```python
from build123d import *

# Parameters (mm, degrees)
SKETCH_1_R      = 2
SKETCH_1_R_2    = 1.65
EXTRUDE_1_DEPTH = 300
FILLET_1_R      = 0.2


with BuildPart() as part:
    # 草图1 → 凸台-拉伸1 (new body)
    with BuildSketch(Plane(origin=(0, 0, 0), x_dir=(1, 0, 0), z_dir=(0, 1, 0))):
        with BuildLine():
            Line((-9.5, 10), (-2.15, 10))
            Line((-2.15, 10), (-2.15, 8.7))
            Line((-2.15, 8.7), (-4, 8.7))
            Line((-4, 8.7), (-4, 4.7))
            Line((-4, 4.7), (-2.15, 4.7))
            Line((-2.15, 4.7), (-2.15, 2.9))
            Line((-2.15, 2.9), (0, 2.9))
            Line((0, 2.9), (2.15, 2.9))
            Line((2.15, 2.9), (2.15, 4.7))
            Line((2.15, 4.7), (4, 4.7))
            Line((4, 4.7), (4, 8.7))
            Line((4, 8.7), (2.15, 8.7))
            Line((2.15, 8.7), (2.15, 10))
            Line((2.15, 10), (9.5, 10))
            ThreePointArc((9.5, 10), (9.853553391, 9.853553391), (10, 9.5))
            Line((10, 9.5), (10, 2.15))
            Line((10, 2.15), (8.7, 2.15))
            Line((8.7, 2.15), (8.7, 4))
            Line((8.7, 4), (4.7, 4))
            Line((4.7, 4), (4.7, 2.15))
            Line((4.7, 2.15), (2.9, 2.15))
            Line((2.9, 2.15), (2.9, 0))
            Line((2.9, 0), (2.9, -2.15))
            Line((2.9, -2.15), (4.7, -2.15))
            Line((4.7, -2.15), (4.7, -4))
            Line((4.7, -4), (8.7, -4))
            Line((8.7, -4), (8.7, -2.15))
            Line((8.7, -2.15), (10, -2.15))
            Line((10, -2.15), (10, -9.5))
            ThreePointArc((10, -9.5), (9.853553391, -9.853553391), (9.5, -10))
            Line((9.5, -10), (2.15, -10))
            Line((2.15, -10), (2.15, -8.7))
            Line((2.15, -8.7), (4, -8.7))
            Line((4, -8.7), (4, -4.7))
            Line((4, -4.7), (2.15, -4.7))
            Line((2.15, -4.7), (2.15, -2.9))
            Line((2.15, -2.9), (0, -2.9))
            Line((0, -2.9), (-2.15, -2.9))
            Line((-2.15, -2.9), (-2.15, -4.7))
            Line((-2.15, -4.7), (-4, -4.7))
            Line((-4, -4.7), (-4, -8.7))
            Line((-4, -8.7), (-2.15, -8.7))
            Line((-2.15, -8.7), (-2.15, -10))
            Line((-2.15, -10), (-9.5, -10))
            ThreePointArc((-9.5, -10), (-9.853553391, -9.853553391), (-10, -9.5))
            Line((-10, -9.5), (-10, -2.15))
            Line((-10, -2.15), (-8.7, -2.15))
            Line((-8.7, -2.15), (-8.7, -4))
            Line((-8.7, -4), (-4.7, -4))
            Line((-4.7, -4), (-4.7, -2.15))
            Line((-4.7, -2.15), (-2.9, -2.15))
            Line((-2.9, -2.15), (-2.9, 0))
            Line((-2.9, 0), (-2.9, 2.15))
            Line((-2.9, 2.15), (-4.7, 2.15))
            Line((-4.7, 2.15), (-4.7, 4))
            Line((-4.7, 4), (-8.7, 4))
            Line((-8.7, 4), (-8.7, 2.15))
            Line((-8.7, 2.15), (-10, 2.15))
            Line((-10, 2.15), (-10, 9.5))
            ThreePointArc((-10, 9.5), (-9.853553391, 9.853553391), (-9.5, 10))
        make_face()
        with Locations(Location((-7.1, 7.1, 0), (0, 0, 270))):
            Circle(SKETCH_1_R, mode=Mode.SUBTRACT)
        with Locations(Location((7.1, 7.1, 0), (0, 0, 270))):
            Circle(SKETCH_1_R, mode=Mode.SUBTRACT)
        with Locations(Location((7.1, -7.1, 0), (0, 0, 270))):
            Circle(SKETCH_1_R, mode=Mode.SUBTRACT)
        with Locations(Location((-7.1, -7.1, 0), (0, 0, 270))):
            Circle(SKETCH_1_R, mode=Mode.SUBTRACT)
        with Locations(Location((0, 0, 0), (0, 0, 270))):
            Circle(SKETCH_1_R_2, mode=Mode.SUBTRACT)
    extrude(amount=EXTRUDE_1_DEPTH)

    # 圆角1
    fillet_1_edges = [part.edges().sort_by_distance(p)[0] for p in [
        (8.7, 150, 2.15),
        (10, 150, 2.15),
        (2.15, 150, 10),
        (2.15, 150, 8.7),
        (4, 150, 8.7),
        (4, 150, 4.7),
        (2.15, 150, 4.7),
        (2.15, 150, 2.9),
        (-2.15, 150, 2.9),
        (-2.15, 150, 4.7),
        (-4, 150, 4.7),
        (-4, 150, 8.7),
        (-2.15, 150, 8.7),
        (-2.15, 150, 10),
        (-10, 150, 2.15),
        (-8.7, 150, 2.15),
        (-8.7, 150, 4),
        (-4.7, 150, 4),
        (-4.7, 150, 2.15),
        (-2.9, 150, 2.15),
        (-2.9, 150, -2.15),
        (-4.7, 150, -2.15),
        (-4.7, 150, -4),
        (-8.7, 150, -4),
        (-8.7, 150, -2.15),
        (-10, 150, -2.15),
        (-2.15, 150, -10),
        (-2.15, 150, -8.7),
        (-4, 150, -8.7),
        (-4, 150, -4.7),
        (-2.15, 150, -4.7),
        (-2.15, 150, -2.9),
        (2.15, 150, -2.9),
        (2.15, 150, -4.7),
        (4, 150, -4.7),
        (4, 150, -8.7),
        (2.15, 150, -8.7),
        (2.15, 150, -10),
        (10, 150, -2.15),
        (8.7, 150, -2.15),
        (8.7, 150, -4),
        (4.7, 150, -4),
        (4.7, 150, -2.15),
        (2.9, 150, -2.15),
        (2.9, 150, 2.15),
        (4.7, 150, 2.15),
        (4.7, 150, 4),
        (8.7, 150, 4),
    ]]
    fillet(fillet_1_edges, radius=FILLET_1_R)


solid = part.part
```
Could you check a few things on this model? Use its own coordinates, in mm. Round coordinates to 2 decimals unless told otherwise and drop trailing zeros. One line per question, with ' | ' between items. Start each with the question number.
(1) For P1, Ø2, axis at y = 148.5, z = 1, coming from the +X side, with a flat end and sliding along its axis, tell me the tip position at first contact or that it passes through.
(2) Suppose I cut it at A-A on y = 247. Count the separate pieces of the cut face and the enclosed holes in it, then the cut area to 3 significant figures.
(3) Please list where these lines run through material, in increasing order: line 1 along Z through (x, y) = (-7.25, 200.5); line 2 along X through (y, z) = (160, -7.1); line 3 along X through (y, z) = (171.5, -3.25).
Geometry results:
1) P1: x = 2.91
2) separate pieces: 1 | enclosed holes: 5 | area: 160 mm²
3) line 1: -10 to -9.09, -5.11 to -4, 4 to 5.11, 9.09 to 10 | line 2: -10 to -9.1, -5.1 to -4, 4 to 5.1, 9.1 to 10 | line 3: -10 to -8.7, -4.7 to -2.15, 2.15 to 4.7, 8.7 to 10
